The listing builds one solid part. Answer for the finished solid, in the listing's coordinates (mm). A direction names the side the tool comes from. Give positions to 0.01 mm unless a question says otherwise; leave off trailing zeros. Loops run counter-clockwise (first coordinate to the right, second up) from the corner with the lowest first, then second, coordinate; pieces in that order, holes last. Notation, with made-up numbers: (40, -37.5) - (65, -37.5) arc R31 cw to (65, -11.5) - close; hole circle Ø3 at (12.25, -19.75). An arc over 180 degrees is marked (long way). Write item = value, one per line. Start each with the question number.
1) Consider probe 1 along Z at (x, y) = (1.75, 64.75); probe 2 along Y at (x, z) = (3.25, 70.5); probe 3 along X at (y, z) = (54.5, 365.5). Determine where each line is inside the solid, lowest interval first.
2) The mould has two halves that part along Z. Classify faces 1 (the flat face through (0, 49.5, 266.8)), 2 (the flat face through (0, 49.5, 265.8)), 3 (the flat face through (0, 49.5, 135.8)): +Z half, -Z half, draft (parallel to the pull), parting line (faces both ways), or undercut.
3) Flat-ended cylindrical pins translate along their axes: P1, Ø3, axis at y = 56.5, z = 224, coming from the +X side; P2, Ø4, axis at x = -5, y = 53, coming from the -Z side; P3, Ø8, axis at y = 46, z = 146.5, coming from the -X side. Find the tip coordinate at first contact, or state that the pin passes through.
4) The part is cut by section B-B on x = 3. Write down the section's boundary in (y, z), plus the area to 3 significant figures.
5) Which of the six approach directions +Z, -Z, +X, -X, +Y, -Y give full straight-line access (tool end or side, diameter ignored) to faces 4 (the cylindrical face through (8.77, 43.81, 266.29)), 5 (the cylindrical face through (2.22, 60.85, 71.71)), 6 (the cylindrical face through (2.22, 60.85, 337.27)), 7 (the flat face through (3, 55, 5.8)), 8 (the flat face through (0, 49.5, 136.8))?
6) The part is cut by section A-A on y = 54.9. Write down the section's boundary in (x, z).
7) The part is cut by section C-C on z = 306.5. Write down the section's boundary in (x, y), plus the area to 3 significant figures.
from build123d import *

# Parameters (mm, degrees)
SKETCH019_R  = 6
PAD010_DEPTH = 400
SKETCH071_R  = 12.5
PAD_DEPTH    = 1
SKETCH_R     = 12.5
PAD011_DEPTH = 1


with BuildPart() as part:
    # Sketch019 → Pad010 (new body)
    with BuildSketch(Plane.XY):
        Circle(SKETCH019_R)
    extrude(amount=-PAD010_DEPTH)

    # Sketch071 (on Face2 of Pad010) → Pad (join)
    with BuildSketch(Plane.XY.offset(-270)):
        Circle(SKETCH071_R)
    extrude(amount=PAD_DEPTH)

    # Sketch (on Face2 of Pad) → Pad011 (join)
    with BuildSketch(Plane.XY.offset(-140)):
        Circle(SKETCH_R)
    extrude(amount=PAD011_DEPTH)


with BuildPart() as part_1:
    # Body007 placement: moved
    add(part.part.moved(Location((3, 54.9, 405.8))))


solid = part_1.part
Answer below:
q1.probe_1 = 135.8 to 136.8, 265.8 to 266.8
q1.probe_2 = 48.91 to 60.89
q1.probe_3 = -2.99 to 8.99
q2.face_1 = +Z half
q2.face_2 = undercut
q2.face_3 = -Z half
q3.P1 = 9
q3.P2 = 135.8
q3.P3 = -0.46
q4.outline = (42.4, 135.8) - (48.9, 135.8) - (48.9, 5.8) - (60.9, 5.8) - (60.9, 135.8) - (67.4, 135.8) - (67.4, 136.8) - (60.9, 136.8) - (60.9, 265.8) - (67.4, 265.8) - (67.4, 266.8) - (60.9, 266.8) - (60.9, 405.8) - (48.9, 405.8) - (48.9, 266.8) - (42.4, 266.8) - (42.4, 265.8) - (48.9, 265.8) - (48.9, 136.8) - (42.4, 136.8) - close
q4.area = 4,830 mm2
q5.face_4 = +Z, -Z
q5.face_5 = -Z
q5.face_6 = +Z
q5.face_7 = -Z, +X, -X, +Y, -Y
q5.face_8 = none
q6.outline = (-9.5, 135.8) - (-3, 135.8) - (-3, 5.8) - (9, 5.8) - (9, 135.8) - (15.5, 135.8) - (15.5, 136.8) - (9, 136.8) - (9, 265.8) - (15.5, 265.8) - (15.5, 266.8) - (9, 266.8) - (9, 405.8) - (-3, 405.8) - (-3, 266.8) - (-9.5, 266.8) - (-9.5, 265.8) - (-3, 265.8) - (-3, 136.8) - (-9.5, 136.8) - close
q7.outline = circle Ø12 at (3, 54.9)
q7.area = 113 mm2
